For this review, take the finished solid that the model builds, in its own axes (mm). Face numbers are marked on the shaded views. A direction names the side the tool comes from. Coordinates: 2 decimals unless noted, no trailing zeros. Order: outer loops, then holes, each group sorted by start corner. A loop starts at its lowest first (then second) coordinate and runs counter-clockwise, first axis right, second up. Notation, with made-up numbers: M -33,-14.75 L 4,-14.75 A10 ccw 4,0.25 Z; hole C 7,53.25 d10. An arc over 180 degrees is marked long. Use CSV: the item, a comma, the result in double quotes.
```python
from build123d import *

# Parameters (mm, degrees)
F1_DEPTH = 1132
F2_W     = 141.117851
F2_H     = 4
F3_DEPTH = 35.318025


with BuildPart() as f1:
    # F0 (on Front) → F1 (new body)
    with BuildSketch(Plane.XZ):
        with BuildLine():
            Line((119.964918, 0), (0, 0))
            Line((0, 0), (0, -4))
            Line((0, -4), (120.314873, -4))
            Line((120.314873, -4), (143, 0))
            Line((143, 0), (296.475341, 0))
            ThreePointArc((296.475341, 0), (301.475473, -1.516773), (304.790256, -5.555849))
            Line((304.790256, -5.555849), (314.695518, -29.469266))
            Line((314.695518, -29.469266), (315.460885, -31.317025))
            Line((315.460885, -31.317025), (319.156403, -29.786292))
            Line((319.156403, -29.786292), (308.485775, -4.025115))
            ThreePointArc((308.485775, -4.025115), (303.697754, 1.809105), (296.475341, 4))
            Line((296.475341, 4), (142.650045, 4))
            Line((142.650045, 4), (119.964918, 0))
        make_face()
    extrude(amount=-F1_DEPTH)

    # F2 (on face) → F3 (cut, through all)
    with BuildSketch(Plane.XY.offset(4)):
        with Locations((263.55897, 66)):
            Rectangle(F2_W, F2_H)
        with Locations((263.55897, 316)):
            Rectangle(F2_W, F2_H)
        with Locations((263.55897, 566)):
            Rectangle(F2_W, F2_H)
        with Locations((263.55897, 816)):
            Rectangle(F2_W, F2_H)
        with Locations((263.55897, 1066)):
            Rectangle(F2_W, F2_H)
    extrude(amount=-F3_DEPTH, mode=Mode.SUBTRACT)


solid = f1.part
```
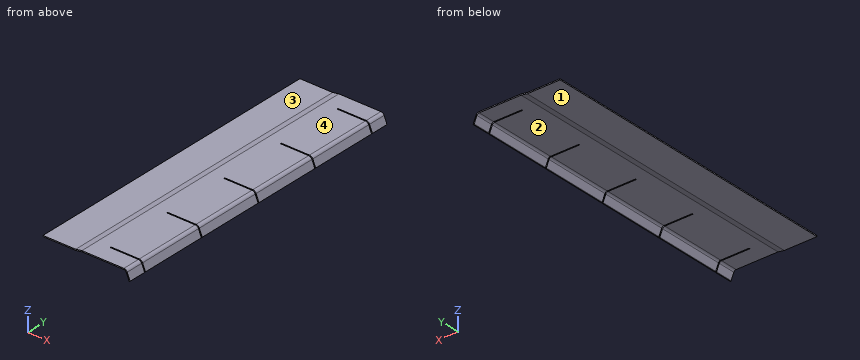
Item 1: Add section A-A on z = -13. State the section outline as (x, y) points, and give its area (3 significant figures).
Solutions:
outline,"M 307.87,0 L 312.2,0 L 312.2,64 L 307.87,64 Z; M 307.87,68 L 312.2,68 L 312.2,314 L 307.87,314 Z; M 307.87,318 L 312.2,318 L 312.2,564 L 307.87,564 Z; M 307.87,568 L 312.2,568 L 312.2,814 L 307.87,814 Z; M 307.87,818 L 312.2,818 L 312.2,1064 L 307.87,1064 Z; M 307.87,1068 L 312.2,1068 L 312.2,1132 L 307.87,1132 Z"
area,"4,810 mm^2"
Item 2: Clearance check with flat-ended pins moving along their axes: pin 1 Ø10 at (x, y) = (139, 613.5) entering from -Z; pin 2 Ø1.2 at (y, z) = (565.5, 1) entering from +X; pin 3 Ø17.5 at (x, z) = (242, -11) entering from +Y (3 decimals); pin 4 Ø17.5 at (x, z) = (227, -8) entering from -Y. State where each tip first meets the part, or that it passes through.
Solutions:
pin 1,"z = -1.59"
pin 2,"x = 193"
pin 3,"through"
pin 4,"y = 0"
Item 3: Add section B-B on y = 599. State the section outline as (x, z) points, and give its area (3 significant figures).
Solutions:
outline,"M 0,-4 L 120.31,-4 L 143,0 L 296.48,0 A9 cw 304.79,-5.56 L 315.46,-31.32 L 319.16,-29.79 L 308.49,-4.03 A13 ccw 296.48,4 L 142.65,4 L 119.96,0 L 0,0 Z"
area,"1,350 mm^2"
Item 4: To check wall thickness, follow line 1 along Y through (x, z) = (281, 1); line 2 along Z through (x, y) = (96, 659); line 3 along Z through (x, y) = (215, 185). State the ranges of each line that lie inside material, in increasing order. Write a range as [from, to].
Solutions:
line 1,"[0, 64], [68, 314], [318, 564], [568, 814], [818, 1064], [1068, 1132]"
line 2,"[-4, 0]"
line 3,"[0, 4]"
Item 5: Draft analysis for pull direction X (two halves, no side actions). For the marked faces 1 and 2, state which applies: released by +X, released by -X, zero draft, split by the parting line, or undercut.
Solutions:
face 1,"zero draft"
face 2,"undercut"
Item 6: For the marked faces 3 and 4, list the 3-axis set-ups (+Z, -Z, +X, -X, +Y, -Y) from which the entire face can be reached by the end or side of a thin tool; tool diameter is ignored.
Solutions:
face 3,"+Z, -X, +Y, -Y"
face 4,"+Z, +X, -X, +Y, -Y"
Item 7: Add section C-C on x = 100.5. State the section outline as (y, z) points, and give its area (3 significant figures).
Solutions:
outline,"M 0,-4 L 1132,-4 L 1132,0 L 0,0 Z"
area,"4,530 mm^2"
